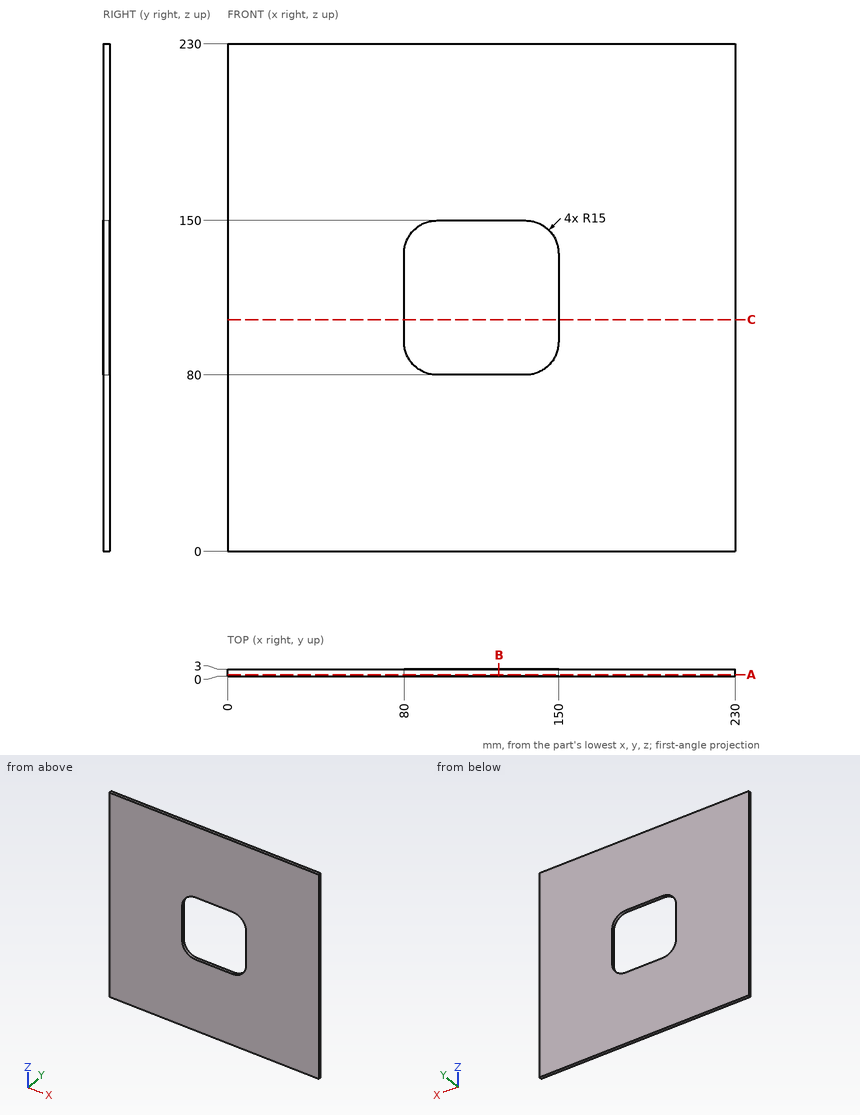
The drawing under review shows one solid part. Ordinate dimensions are in mm from its lowest x, y, z. Coordinates: 2 decimals unless noted, no trailing zeros. Loops run counter-clockwise (first coordinate to the right, second up) from the corner with the lowest first, then second, coordinate; pieces in that order, holes last. Notation, with made-up numbers: (-18, 34) - (35, 34) arc R15 cw to (35, 53) - close; hole circle Ø11 at (45, 40). An arc over 180 degrees is marked (long way). Use CSV: the item, a comma, the result in double quotes. Start each with the question number.
1. Add section A-A on y = 0.65. Give the boundary of the cut face in (x, z).
2. Clearance check with a flat-ended pin moving along its axis: pin 1 (6 mm diameter, centred on x = 50.5, z = 198.5, fed in from -Y). State where the tip first meets the part, or that it passes through.
3. Add section C-C on z = 105. Give the boundary of the cut face in (x, y), plus the area to 3 significant figures.
4. Add section B-B on x = 123. Give the boundary of the cut face in (y, z), plus the area to 3 significant figures.
5. To check wall thickness, follow probe 1 along X at (y, z) = (1.45, 133.5); probe 2 along Z at (x, y) = (84.5, 2.25). State the ranges of each line that lie inside material, in increasing order.
Resolved:
1,outline,"(0, 0) - (230, 0) - (230, 230) - (0, 230) - close; hole (80, 95) arc R15 ccw to (95, 80) - (135, 80) arc R15 ccw to (150, 95) - (150, 135) arc R15 ccw to (135, 150) - (95, 150) arc R15 ccw to (80, 135) - close"
2,pin 1,"y = 0"
3,outline,"(0, 0) - (80, 0) - (80, 3) - (0, 3) - close; (150, 0) - (230, 0) - (230, 3) - (150, 3) - close"
3,area,"480 mm2"
4,outline,"(0, 0) - (3, 0) - (3, 80) - (0, 80) - close; (0, 150) - (3, 150) - (3, 230) - (0, 230) - close"
4,area,"480 mm2"
5,probe 1,"0 to 80, 150 to 230"
5,probe 2,"0 to 84.29, 145.71 to 230"
